Read the model definition and answer for the solid it produces. Units are mm, in the model's axes. A direction names the side the tool comes from. Coordinates: 2 decimals unless noted, no trailing zeros. Order: outer loops, then holes, each group sorted by start corner. A loop starts at its lowest first (then second) coordinate and runs counter-clockwise, first axis right, second up. Notation, with made-up numbers: (49.5, 34) -> (108.5, 34) arc R31 cw to (108.5, 72) -> close; hole circle Ø11 at (25, -13). An arc over 180 degrees is marked (long way). Answer as a JSON object with one key per item and string values. Group by question number.
1) Section C-C on z = 8.75 is taken. Determine the outline of the cut face in (x, y), and give its area (3 significant figures).
2) Consider L1, parallel to Y at x = 19, z = 7.75; L2, parallel to Y at x = 15, z = 1.4 (3 decimals); L3, parallel to Z at x = 9, y = -5. Determine where each line is inside the solid, lowest interval first.
3) Section B-B on x = 43 is taken. Determine the outline of the cut face in (y, z) (3 decimals), and give its area (4 significant figures).
4) Determine the mould class of faces 1 (the cylindrical face through (40.6, -17.8, 5.5)), 2 (the flat face through (0, -16, 7)), 3 (the flat face through (29, 5, 6)) for opening direction Y: released by +Y, released by -Y, zero draft, split by the parting line, or undercut.
5) Section D-D on x = 31.5 is taken. Determine the outline of the cut face in (y, z), and give its area (4 significant figures).
6) Given pin 1 (2.5 mm diameter, centred on x = 3, y = -11.5, fed in from +Z); pin 2 (9.5 mm diameter, centred on x = 34, y = -11.5, fed in from +Z); pin 3 (5 mm diameter, centred on x = 3.5, y = -16, fed in from -Z), each flat-ended and moving along its own axis, determine where each tip first touches the part or whether it passes through.
7) Section A-A on y = -16 is taken. Determine the outline of the cut face in (x, z) (3 decimals).
8) A tool of negligible diameter and unlimited length cuts with its end or side. For faces 4 (the flat face through (5, -16, 8)), 5 (the flat face through (5, -16, 3.25)), 6 (the cylindrical face through (15.75, -17.44, 2.03)), 7 (the flat face through (28.59, 2.53, 12.15)), 8 (the flat face through (2, -16, 10)), from which of +Z, -Z, +X, -X, +Y, -Y can it reach the whole face along a straight path? Write none if from no direction.
from build123d import *

# Parameters (mm, degrees)
ESQUISSE1_W                  = 58
ESQUISSE1_H                  = 32
BOSS_EXTRU_1_DEPTH           = 7
ESQUISSE2_W                  = 5
ESQUISSE2_H                  = 32
BOSS_EXTRU_3_DEPTH           = 3
ESQUISSE3_W                  = 5
ESQUISSE3_H                  = 32
BOSS_EXTRU_4_DEPTH           = 5
ENL_V_MAT_EXTRU_1_DEPTH      = 33
ESQUISSE6_R                  = 1.625
ENL_V_MAT_EXTRU_2_DEPTH      = 8
ESQUISSE8_R                  = 3
ENL_V_MAT_EXTRU_4_DEPTH      = 3
ESQUISSE7_W                  = 10.25
ESQUISSE7_H                  = 3.25
ENL_V_MAT_EXTRU_3_DEPTH      = 10
ENL_V_MAT_EXTRU_3_DEPTH_BACK = 50
ESQUISSE9_W                  = 58
ESQUISSE9_H                  = 5
BOSS_EXTRU_5_DEPTH           = 12
BOSS_EXTRU_6_DEPTH           = 58
ESQUISSE12_W                 = 10.25
ESQUISSE12_H                 = 5
ENL_V_MAT_EXTRU_5_DEPTH      = 3.25


with BuildPart() as part:
    # Esquisse1 → Boss.-Extru.1 (new body)
    with BuildSketch(Plane.XY):
        with Locations((29, -16)):
            Rectangle(ESQUISSE1_W, ESQUISSE1_H)
    extrude(amount=BOSS_EXTRU_1_DEPTH)

    # Esquisse2 → Boss.-Extru.3 (add)
    with BuildSketch(Plane.XY.offset(7)):
        with Locations((2.5, -16)):
            Rectangle(ESQUISSE2_W, ESQUISSE2_H)
    extrude(amount=BOSS_EXTRU_3_DEPTH)

    # Esquisse3 → Boss.-Extru.4 (add)
    with BuildSketch(Plane.XY.offset(7)):
        with Locations((55.5, -16)):
            Rectangle(ESQUISSE3_W, ESQUISSE3_H)
    extrude(amount=BOSS_EXTRU_4_DEPTH)

    # Esquisse4 → Enlèv. mat.-Extru.1 (cut, through all)
    with BuildSketch(Plane.XZ.offset(32)):
        Polygon((0, 10), (58, 12), (0, 12), align=None)
    extrude(amount=-ENL_V_MAT_EXTRU_1_DEPTH, mode=Mode.SUBTRACT)

    # Esquisse6 → Enlèv. mat.-Extru.2 (cut, through all)
    with BuildSketch(Plane.XY.offset(7)):
        with Locations((43, -16)):
            Circle(ESQUISSE6_R)
        with Locations((15, -16)):
            Circle(ESQUISSE6_R)
    extrude(amount=-ENL_V_MAT_EXTRU_2_DEPTH, mode=Mode.SUBTRACT)

    # Esquisse8 → Enlèv. mat.-Extru.4 (cut)
    with BuildSketch(Plane.XY.offset(7)):
        with Locations((15, -16)):
            Circle(ESQUISSE8_R)
        with Locations((43, -16)):
            Circle(ESQUISSE8_R)
    extrude(amount=-ENL_V_MAT_EXTRU_4_DEPTH, mode=Mode.SUBTRACT)

    # Esquisse7 → Enlèv. mat.-Extru.3 (cut, two sides)
    with BuildSketch(Plane.XZ.offset(32)) as enl_v_mat_extru_3_sk:
        with Locations((5.125, 1.625)):
            Rectangle(ESQUISSE7_W, ESQUISSE7_H)
    extrude(amount=ENL_V_MAT_EXTRU_3_DEPTH, mode=Mode.SUBTRACT)
    extrude(enl_v_mat_extru_3_sk.sketch, amount=-ENL_V_MAT_EXTRU_3_DEPTH_BACK, mode=Mode.SUBTRACT)

    # Esquisse9 → Boss.-Extru.5 (add)
    with BuildSketch(Plane.XY):
        with Locations((29, 2.5)):
            Rectangle(ESQUISSE9_W, ESQUISSE9_H)
        with Locations((29, -34.5)):
            Rectangle(ESQUISSE9_W, ESQUISSE9_H)
    extrude(amount=BOSS_EXTRU_5_DEPTH)

    # Esquisse10 → Boss.-Extru.6 (add, through all)
    with BuildSketch(Plane.ZY):
        Polygon((12, 5), (12.3, 5), (12, 0), align=None)
        Polygon((12, -32), (12, -37), (12.3, -37), align=None)
    extrude(amount=-BOSS_EXTRU_6_DEPTH)

    # Esquisse12 → Enlèv. mat.-Extru.5 (cut)
    with BuildSketch(Plane(origin=(0, 0, 0), x_dir=(-1, 0, 0), z_dir=(0, 0, -1))):
        with Locations((-5.125, -34.5)):
            Rectangle(ESQUISSE12_W, ESQUISSE12_H)
        with Locations((-5.125, 2.5)):
            Rectangle(ESQUISSE12_W, ESQUISSE12_H)
    extrude(amount=-ENL_V_MAT_EXTRU_5_DEPTH, mode=Mode.SUBTRACT)


solid = part.part
Worked answers:
{
 "1": {"outline": "(0, -37) -> (58, -37) -> (58, 5) -> (0, 5) -> close; hole (5, -32) -> (53, -32) -> (53, 0) -> (5, 0) -> close", "area": "900 mm²"},
 "2": {"L1": "y = -37 to -32, 0 to 5", "L2": "y = -37 to -17.625, -14.375 to 5", "L3": "z = 3.25 to 7"},
 "3": {"outline": "(-37, 0) -> (-17.625, 0) -> (-17.625, 4) -> (-19, 4) -> (-19, 7) -> (-32, 7) -> (-32, 12) -> (-37, 12.3) -> close; (-14.375, 0) -> (5, 0) -> (5, 12.3) -> (0, 12) -> (0, 7) -> (-13, 7) -> (-13, 4) -> (-14.375, 4) -> close", "area": "314.5 mm²"},
 "4": {"face 1": "undercut", "face 2": "zero draft", "face 3": "released by +Y"},
 "5": {"outline": "(-37, 0) -> (5, 0) -> (5, 12.3) -> (0, 12) -> (0, 7) -> (-32, 7) -> (-32, 12) -> (-37, 12.3) -> close", "area": "345.5 mm²"},
 "6": {"pin 1": "stops at z = 10", "pin 2": "stops at z = 7", "pin 3": "stops at z = 3.25"},
 "7": {"outline": "(0, 3.25) -> (10.25, 3.25) -> (10.25, 0) -> (13.375, 0) -> (13.375, 4) -> (12, 4) -> (12, 7) -> (5, 7) -> (5, 10) -> (0, 10) -> close; (16.625, 0) -> (41.375, 0) -> (41.375, 4) -> (40, 4) -> (40, 7) -> (18, 7) -> (18, 4) -> (16.625, 4) -> close; (44.625, 0) -> (58, 0) -> (58, 12) -> (53, 11.828) -> (53, 7) -> (46, 7) -> (46, 4) -> (44.625, 4) -> close"},
 "8": {"face 4": "+Z", "face 5": "-Z, -X, +Y, -Y", "face 6": "+Z, -Z", "face 7": "+Z, +X, -X", "face 8": "+Z, -X"}
}
